Verification items for the finished model (mm, model axes). Face numbers are marked on the shaded views. A direction names the side the tool comes from. Coordinates: 2 decimals unless noted, no trailing zeros. Order: outer loops, then holes, each group sorted by start corner. A loop starts at its lowest first (then second) coordinate and runs counter-clockwise, first axis right, second up. Notation, with made-up numbers: M 3,65.5 L 13,65.5 A28 cw 13,99.5 Z; hole C 65,-31 d2. An arc over 180 degrees is marked long. Return JSON: item names as keys, results as strings. Group by question number.
1. Material ranges on line 1 along X through (y, z) = (-4, 0); line 2 along Y through (x, z) = (17.75, 0); line 3 along Z through (x, y) = (20, -4.3), recorded low to high.
2. Section check D-D, the plane x = 20. Record the cut outline in (y, z).
3. Mould release check, pull along Y, two halves, no side actions. Record for the marked faces 1, 2 and 3: +Y half, -Y half, draft (parallel to the pull), parting line (faces both ways), or undercut.
4. Section check B-B, the plane y = 0. Record the cut outline in (x, z) (3 decimals).
5. Gauge pin test, flat ends, axial feed: pin 1 (5 mm diameter, centred on x = 18, z = -5.5, fed in from +Y); pin 2 (3 mm diameter, centred on x = 17.5, z = 6.5, fed in from -Y); pin 3 (1 mm diameter, centred on x = 18.5, z = 0, fed in from +Y); pin 4 (4.5 mm diameter, centred on y = 0, z = 0, fed in from -X). Record the tip position at first contact, or that the pin passes through.
6. Set-up check for the marked faces 4, 5 and 6: record each of +Z, -Z, +X, -X, +Y, -Y from which the full face is reachable in a straight line by a thin tool's end or side.
7. Section check A-A, the plane z = 0. Record the cut outline in (x, y) (3 decimals), plus the area to 3 significant figures.
8. Section check C-C, the plane x = 14.5. Record the cut outline in (y, z), plus the area to 3 significant figures.
```python
from build123d import *

# Parameters (mm, degrees)
TAP_DRILL_FOR_M3X0_5_TAP1_REACH  = 21.005
TAP_DRILL_FOR_M3X0_5_TAP1_BORE_R = 1.3


with BuildPart() as part:
    # Sketch1 → Revolve1 (revolve)
    with BuildSketch(Plane(origin=(0, 0, 0), x_dir=(-1, 0, 0), z_dir=(0, 0, -1)), mode=Mode.PRIVATE) as revolve1_sk:
        Polygon((-22.5, 3.5), (-22.5, 2.5), (-12.5, 2.5), (-12.5, 4.9), (-11.71, 6.053145161), (-15.64, 8.715), (-17.5, 6), (-22, 6), (-22, 3.5), align=None)
    revolve(revolve1_sk.sketch.rotate(Axis((22.5, 0, 0), (-1, 0, 0)), 270), axis=Axis((22.5, 0, 0), (-1, 0, 0)))

    # Tap Drill for M3x0.5 Tap1 bore (on position points) → Tap Drill for M3x0.5 Tap1 (cut, up to next)
    with BuildSketch(Plane(origin=(20, -6, 0), x_dir=(0, 0, -1), z_dir=(0, -1, 0)), mode=Mode.PRIVATE) as tap_drill_for_m3x0_5_tap1_sk1:
        Circle(TAP_DRILL_FOR_M3X0_5_TAP1_BORE_R)
    tap_drill_for_m3x0_5_tap1_tool1 = extrude(tap_drill_for_m3x0_5_tap1_sk1.sketch, amount=-TAP_DRILL_FOR_M3X0_5_TAP1_REACH, mode=Mode.PRIVATE) & part.part
    add(tap_drill_for_m3x0_5_tap1_tool1.solids().sort_by_distance((20, -6, 0))[0], mode=Mode.SUBTRACT)


solid = part.part
```
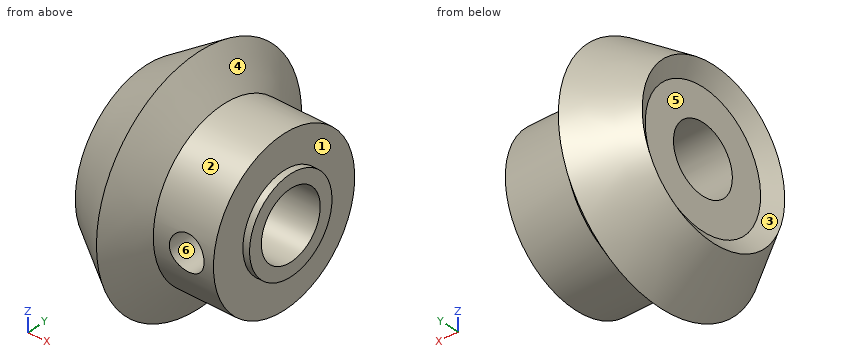
Answers follow:
{
 "1": {"line 1": "12.5 to 18.7, 21.3 to 22", "line 2": "-6 to -2.5, 2.5 to 6", "line 3": "-4.18 to -1.3, 1.3 to 4.18"},
 "2": {"outline": "M -5.86,-1.3 A6 ccw long -5.86,1.3 L -2.14,1.3 A2.5 cw long -2.14,-1.3 Z"},
 "3": {"face 1": "draft", "face 2": "parting line", "face 3": "undercut"},
 "4": {"outline": "M 11.71,-6.053 L 15.64,-8.715 L 17.5,-6 L 22,-6 L 22,-3.5 L 22.5,-3.5 L 22.5,-2.5 L 12.5,-2.5 L 12.5,-4.9 Z; M 11.71,6.053 L 12.5,4.9 L 12.5,2.5 L 22.5,2.5 L 22.5,3.5 L 22,3.5 L 22,6 L 17.5,6 L 15.64,8.715 Z"},
 "5": {"pin 1": "y = 7.36", "pin 2": "y = -5.42", "pin 3": "y = 6", "pin 4": "through"},
 "6": {"face 4": "+X", "face 5": "-X", "face 6": "-Y"},
 "7": {"outline": "M 11.71,-6.053 L 15.64,-8.715 L 17.5,-6 L 18.7,-6 L 18.7,-2.5 L 12.5,-2.5 L 12.5,-4.9 Z; M 11.71,6.053 L 12.5,4.9 L 12.5,2.5 L 22.5,2.5 L 22.5,3.5 L 22,3.5 L 22,6 L 17.5,6 L 15.64,8.715 Z; M 21.3,-6 L 22,-6 L 22,-3.5 L 22.5,-3.5 L 22.5,-2.5 L 21.3,-2.5 Z", "area": "75.2 mm^2"},
 "8": {"outline": "C 0,0 d15.89; hole C 0,0 d5", "area": "179 mm^2"}
}
